Check sheet for the modelled part. Datum: model origin and axes. Units: mm. A direction names the side the tool comes from. Give positions to 0.01 mm unless a question says otherwise; leave off trailing zeros. Order: outer loops, then holes, each group sorted by start corner. A loop starts at its lowest first (then second) coordinate and runs counter-clockwise, first axis right, second up. Notation, with made-up numbers: M 61.25,36 L 103.25,36 A14 ccw 103.25,50 Z; hole C 64.5,84 d2. An arc over 180 degrees is marked long. One line per question, with ' | ' between items. Start each with the question number.
```python
from build123d import *

# Parameters (mm, degrees)
F0_DEPTH = 152.4


with BuildPart() as f0:
    # F1 (on Right) → F0 (new body)
    with BuildSketch(Plane.YZ):
        with BuildLine():
            ThreePointArc((75.710623, -8.622155), (76.077557, -4.318016), (76.2, 0))
            ThreePointArc((76.2, 0), (76.077557, 4.318016), (75.710623, 8.622155))
            ThreePointArc((75.710623, 8.622155), (75.261852, 11.920306), (74.669474, 15.195713))
            ThreePointArc((74.669474, 15.195713), (72.470507, 23.547095), (69.340689, 31.596025))
            ThreePointArc((69.340689, 31.596025), (67.894697, 34.594076), (66.319156, 37.526118))
            ThreePointArc((66.319156, 37.526118), (61.647095, 44.789236), (56.183205, 51.477057))
            ThreePointArc((56.183205, 51.477057), (53.881537, 53.881537), (51.477057, 56.183205))
            ThreePointArc((51.477057, 56.183205), (44.789236, 61.647095), (37.526118, 66.319156))
            ThreePointArc((37.526118, 66.319156), (34.594076, 67.894697), (31.596025, 69.340689))
            ThreePointArc((31.596025, 69.340689), (23.547095, 72.470507), (15.195713, 74.669474))
            ThreePointArc((15.195713, 74.669474), (11.920306, 75.261852), (8.622155, 75.710623))
            ThreePointArc((8.622155, 75.710623), (0, 76.2), (-8.622155, 75.710623))
            ThreePointArc((-8.622155, 75.710623), (-11.920306, 75.261852), (-15.195713, 74.669474))
            ThreePointArc((-15.195713, 74.669474), (-23.547095, 72.470507), (-31.596025, 69.340689))
            ThreePointArc((-31.596025, 69.340689), (-34.594076, 67.894697), (-37.526118, 66.319156))
            ThreePointArc((-37.526118, 66.319156), (-44.789236, 61.647095), (-51.477057, 56.183205))
            ThreePointArc((-51.477057, 56.183205), (-53.881537, 53.881537), (-56.183205, 51.477057))
            ThreePointArc((-56.183205, 51.477057), (-61.647095, 44.789236), (-66.319156, 37.526118))
            ThreePointArc((-66.319156, 37.526118), (-67.894697, 34.594076), (-69.340689, 31.596025))
            ThreePointArc((-69.340689, 31.596025), (-72.470507, 23.547095), (-74.669474, 15.195713))
            ThreePointArc((-74.669474, 15.195713), (-75.261852, 11.920306), (-75.710623, 8.622155))
            ThreePointArc((-75.710623, 8.622155), (-76.2, 0), (-75.710623, -8.622155))
            ThreePointArc((-75.710623, -8.622155), (-75.261852, -11.920306), (-74.669474, -15.195713))
            ThreePointArc((-74.669474, -15.195713), (-72.470507, -23.547095), (-69.340689, -31.596025))
            ThreePointArc((-69.340689, -31.596025), (-67.894697, -34.594076), (-66.319156, -37.526118))
            ThreePointArc((-66.319156, -37.526118), (-61.647095, -44.789236), (-56.183205, -51.477057))
            ThreePointArc((-56.183205, -51.477057), (-53.881537, -53.881537), (-51.477057, -56.183205))
            ThreePointArc((-51.477057, -56.183205), (-44.789236, -61.647095), (-37.526118, -66.319156))
            ThreePointArc((-37.526118, -66.319156), (-34.594076, -67.894697), (-31.596025, -69.340689))
            ThreePointArc((-31.596025, -69.340689), (-23.547095, -72.470507), (-15.195713, -74.669474))
            ThreePointArc((-15.195713, -74.669474), (-11.920306, -75.261852), (-8.622155, -75.710623))
            ThreePointArc((-8.622155, -75.710623), (0, -76.2), (8.622155, -75.710623))
            ThreePointArc((8.622155, -75.710623), (11.920306, -75.261852), (15.195713, -74.669474))
            ThreePointArc((15.195713, -74.669474), (23.547095, -72.470507), (31.596025, -69.340689))
            ThreePointArc((31.596025, -69.340689), (34.594076, -67.894697), (37.526118, -66.319156))
            ThreePointArc((37.526118, -66.319156), (44.789236, -61.647095), (51.477057, -56.183205))
            ThreePointArc((51.477057, -56.183205), (53.881537, -53.881537), (56.183205, -51.477057))
            ThreePointArc((56.183205, -51.477057), (61.647095, -44.789236), (66.319156, -37.526118))
            ThreePointArc((66.319156, -37.526118), (67.894697, -34.594076), (69.340689, -31.596025))
            ThreePointArc((69.340689, -31.596025), (72.470507, -23.547095), (74.669474, -15.195713))
            ThreePointArc((74.669474, -15.195713), (75.261852, -11.920306), (75.710623, -8.622155))
        make_face()
        with BuildLine():
            ThreePointArc((-31.596025, 69.340689), (-23.547095, 72.470507), (-15.195713, 74.669474))
            ThreePointArc((-15.195713, 74.669474), (-20.764473, 78.314179), (-23.898246, 84.185671))
            Line((-23.898246, 84.185671), (-30.149009, 82.154676))
            ThreePointArc((-30.149009, 82.154676), (-29.233108, 75.562553), (-31.596025, 69.340689))
        make_face()
        with BuildLine():
            ThreePointArc((-51.477057, 56.183205), (-44.789236, 61.647095), (-37.526118, 66.319156))
            ThreePointArc((-37.526118, 66.319156), (-43.948599, 68.064635), (-48.743386, 72.680367))
            Line((-48.743386, 72.680367), (-54.060602, 68.817184))
            ThreePointArc((-54.060602, 68.817184), (-51.152451, 62.830731), (-51.477057, 56.183205))
        make_face()
        with BuildLine():
            ThreePointArc((-66.319156, 37.526118), (-61.647095, 44.789236), (-56.183205, 51.477057))
            ThreePointArc((-56.183205, 51.477057), (-62.830731, 51.152451), (-68.817184, 54.060602))
            Line((-68.817184, 54.060602), (-72.680367, 48.743386))
            ThreePointArc((-72.680367, 48.743386), (-68.064635, 43.948599), (-66.319156, 37.526118))
        make_face()
        with BuildLine():
            ThreePointArc((-74.669474, 15.195713), (-72.470507, 23.547095), (-69.340689, 31.596025))
            ThreePointArc((-69.340689, 31.596025), (-75.562553, 29.233108), (-82.154676, 30.149009))
            Line((-82.154676, 30.149009), (-84.185671, 23.898246))
            ThreePointArc((-84.185671, 23.898246), (-78.314179, 20.764473), (-74.669474, 15.195713))
        make_face()
        with BuildLine():
            ThreePointArc((-75.710623, -8.622155), (-76.2, 0), (-75.710623, 8.622155))
            ThreePointArc((-75.710623, 8.622155), (-80.897785, 4.452225), (-87.450296, 3.28622))
            Line((-87.450296, 3.28622), (-87.450296, -3.28622))
            ThreePointArc((-87.450296, -3.28622), (-80.897785, -4.452225), (-75.710623, -8.622155))
        make_face()
        with BuildLine():
            ThreePointArc((-82.154676, -30.149009), (-75.562553, -29.233108), (-69.340689, -31.596025))
            ThreePointArc((-69.340689, -31.596025), (-72.470507, -23.547095), (-74.669474, -15.195713))
            ThreePointArc((-74.669474, -15.195713), (-78.314179, -20.764473), (-84.185671, -23.898246))
            Line((-84.185671, -23.898246), (-82.154676, -30.149009))
        make_face()
        with BuildLine():
            ThreePointArc((-68.817184, -54.060602), (-62.830731, -51.152451), (-56.183205, -51.477057))
            ThreePointArc((-56.183205, -51.477057), (-61.647095, -44.789236), (-66.319156, -37.526118))
            ThreePointArc((-66.319156, -37.526118), (-68.064635, -43.948599), (-72.680367, -48.743386))
            Line((-72.680367, -48.743386), (-68.817184, -54.060602))
        make_face()
        with BuildLine():
            ThreePointArc((-48.743386, -72.680367), (-43.948599, -68.064635), (-37.526118, -66.319156))
            ThreePointArc((-37.526118, -66.319156), (-44.789236, -61.647095), (-51.477057, -56.183205))
            ThreePointArc((-51.477057, -56.183205), (-51.152451, -62.830731), (-54.060602, -68.817184))
            Line((-54.060602, -68.817184), (-48.743386, -72.680367))
        make_face()
        with BuildLine():
            ThreePointArc((-23.898246, -84.185671), (-20.764473, -78.314179), (-15.195713, -74.669474))
            ThreePointArc((-15.195713, -74.669474), (-23.547095, -72.470507), (-31.596025, -69.340689))
            ThreePointArc((-31.596025, -69.340689), (-29.233108, -75.562553), (-30.149009, -82.154676))
            Line((-30.149009, -82.154676), (-23.898246, -84.185671))
        make_face()
        with BuildLine():
            ThreePointArc((3.28622, -87.450296), (4.452225, -80.897785), (8.622155, -75.710623))
            ThreePointArc((8.622155, -75.710623), (0, -76.2), (-8.622155, -75.710623))
            ThreePointArc((-8.622155, -75.710623), (-4.452225, -80.897785), (-3.28622, -87.450296))
            Line((-3.28622, -87.450296), (3.28622, -87.450296))
        make_face()
        with BuildLine():
            ThreePointArc((30.149009, -82.154676), (29.233108, -75.562553), (31.596025, -69.340689))
            ThreePointArc((31.596025, -69.340689), (23.547095, -72.470507), (15.195713, -74.669474))
            ThreePointArc((15.195713, -74.669474), (20.764473, -78.314179), (23.898246, -84.185671))
            Line((23.898246, -84.185671), (30.149009, -82.154676))
        make_face()
        with BuildLine():
            ThreePointArc((54.060602, -68.817184), (51.152451, -62.830731), (51.477057, -56.183205))
            ThreePointArc((51.477057, -56.183205), (44.789236, -61.647095), (37.526118, -66.319156))
            ThreePointArc((37.526118, -66.319156), (43.948599, -68.064635), (48.743386, -72.680367))
            Line((48.743386, -72.680367), (54.060602, -68.817184))
        make_face()
        with BuildLine():
            ThreePointArc((72.680367, -48.743386), (68.064635, -43.948599), (66.319156, -37.526118))
            ThreePointArc((66.319156, -37.526118), (61.647095, -44.789236), (56.183205, -51.477057))
            ThreePointArc((56.183205, -51.477057), (62.830731, -51.152451), (68.817184, -54.060602))
            Line((68.817184, -54.060602), (72.680367, -48.743386))
        make_face()
        with BuildLine():
            ThreePointArc((84.185671, -23.898246), (78.314179, -20.764473), (74.669474, -15.195713))
            ThreePointArc((74.669474, -15.195713), (72.470507, -23.547095), (69.340689, -31.596025))
            ThreePointArc((69.340689, -31.596025), (75.562553, -29.233108), (82.154676, -30.149009))
            Line((82.154676, -30.149009), (84.185671, -23.898246))
        make_face()
        with BuildLine():
            ThreePointArc((75.710623, 8.622155), (76.077557, 4.318016), (76.2, 0))
            ThreePointArc((76.2, 0), (76.077557, -4.318016), (75.710623, -8.622155))
            ThreePointArc((75.710623, -8.622155), (80.897785, -4.452225), (87.450296, -3.28622))
            Line((87.450296, -3.28622), (87.450296, 3.28622))
            ThreePointArc((87.450296, 3.28622), (80.897785, 4.452225), (75.710623, 8.622155))
        make_face()
        with BuildLine():
            ThreePointArc((69.340689, 31.596025), (72.470507, 23.547095), (74.669474, 15.195713))
            ThreePointArc((74.669474, 15.195713), (78.314179, 20.764473), (84.185671, 23.898246))
            Line((84.185671, 23.898246), (82.154676, 30.149009))
            ThreePointArc((82.154676, 30.149009), (75.562553, 29.233108), (69.340689, 31.596025))
        make_face()
        with BuildLine():
            ThreePointArc((56.183205, 51.477057), (61.647095, 44.789236), (66.319156, 37.526118))
            ThreePointArc((66.319156, 37.526118), (68.064635, 43.948599), (72.680367, 48.743386))
            Line((72.680367, 48.743386), (68.817184, 54.060602))
            ThreePointArc((68.817184, 54.060602), (62.830731, 51.152451), (56.183205, 51.477057))
        make_face()
        with BuildLine():
            ThreePointArc((37.526118, 66.319156), (44.789236, 61.647095), (51.477057, 56.183205))
            ThreePointArc((51.477057, 56.183205), (51.152451, 62.830731), (54.060602, 68.817184))
            Line((54.060602, 68.817184), (48.743386, 72.680367))
            ThreePointArc((48.743386, 72.680367), (43.948599, 68.064635), (37.526118, 66.319156))
        make_face()
        with BuildLine():
            ThreePointArc((15.195713, 74.669474), (23.547095, 72.470507), (31.596025, 69.340689))
            ThreePointArc((31.596025, 69.340689), (29.233108, 75.562553), (30.149009, 82.154676))
            Line((30.149009, 82.154676), (23.898246, 84.185671))
            ThreePointArc((23.898246, 84.185671), (20.764473, 78.314179), (15.195713, 74.669474))
        make_face()
        with BuildLine():
            ThreePointArc((-8.622155, 75.710623), (0, 76.2), (8.622155, 75.710623))
            ThreePointArc((8.622155, 75.710623), (4.452225, 80.897785), (3.28622, 87.450296))
            Line((3.28622, 87.450296), (-3.28622, 87.450296))
            ThreePointArc((-3.28622, 87.450296), (-4.452225, 80.897785), (-8.622155, 75.710623))
        make_face()
    extrude(amount=-F0_DEPTH)


solid = f0.part
```
Item 1: Draft check along Y on faces 4 (the face through (-75.13, -68.02, -43.87)), 5 (the face through (-75.133, 78.245, 20.701)), 6 (the face through (-75.133, -75.656, -29.223)). Enter one of: released by +Y, released by -Y, zero draft, split by the parting line, or undercut.
Item 2: Set-up check for faces 1 (the face through (-75.133, -20.701, 78.245)), 2 (the face through (-75.133, 29.223, -75.656)), 3 (the face through (-75.133, -67.916, -34.553)): record each of +Z, -Z, +X, -X, +Y, -Y from which the full face is reachable in a straight line by a thin tool's end or side.
Item 3: Go/stop test with flat-tipped pins: P1, Ø5, axis at x = -55, y = -46, coming from the +Z side; P2, Ø3, axis at x = -64.5, y = -44, coming from the -Z side; P3, Ø1.5, axis at x = -59.5, y = -30, coming from the +Z side. Record where each tip stops, or that it passes through.
Item 4: Scan lines: probe 1 along Y at (x, z) = (-63.5, -80); probe 2 along Z at (x, y) = (-53.5, -78.5); probe 3 along Z at (x, y) = (-15, -15). Record each from-to range of solid material in increasing order. Write a range as [from, to].
Item 5: Section check B-B, the plane y = 18.5. Record the cut outline in (x, z), then the cut area to 3 significant figures.
Item 6: Section check A-A, the plane z = -11.5. Record the cut outline in (x, y), then the cut area to 3 significant figures.
Reported:
1) face 4: released by -Y | face 5: released by +Y | face 6: undercut
2) face 1: +Z, +X, -X | face 2: +X, -X | face 3: +X, -X, -Y
3) P1: stops at z = 72.3 | P2: stops at z = -69.09 | P3: stops at z = 82.45
4) probe 1: y = [-29.47, -22.08], [-4.9, 4.9], [22.08, 29.47] | probe 2: z = [-29.22, -20.93], [-5.86, 5.86], [20.93, 29.22] | probe 3: z = [-74.71, 74.71]
5) outline: M -152.4,-76.34 L 0,-76.34 L 0,76.34 L -152.4,76.34 Z | area: 23,300 mm^2
6) outline: M -152.4,-75.33 L 0,-75.33 L 0,75.33 L -152.4,75.33 Z | area: 23,000 mm^2
